```python
from build123d import *

# Parameters (mm, degrees)
F0_W     = 910
F0_H     = 1270
F1_DEPTH = 890
F2_W     = 950
F2_H     = 380
F3_DEPTH = 610
F4_W     = 160
F4_H     = 190
F5_DEPTH = 610


with BuildPart() as f1:
    # F0 (on Top) → F1 (new body)
    with BuildSketch(Plane.XY):
        with Locations((10.50148, 0)):
            Rectangle(F0_W, F0_H)
    extrude(amount=F1_DEPTH)

    # F2 (on face) → F3 (cut)
    with BuildSketch(Plane(origin=(-444.49852, 0, 0), x_dir=(0, -1, 0), z_dir=(-1, 0, 0))):
        with Locations((0, 700)):
            Rectangle(F2_W, F2_H)
    extrude(amount=-F3_DEPTH, mode=Mode.SUBTRACT)

    # F4 (on face) → F5 (cut, through all)
    with BuildSketch(Plane(origin=(-444.49852, 0, 0), x_dir=(0, -1, 0), z_dir=(-1, 0, 0))):
        with Locations((-555, 795)):
            Rectangle(F4_W, F4_H)
        with Locations((555, 795)):
            Rectangle(F4_W, F4_H)
    extrude(amount=-F5_DEPTH, mode=Mode.SUBTRACT)


solid = f1.part
```
Check sheet for the modelled part. Datum: model origin and axes. Units: mm. A direction names the side the tool comes from. Give positions to 0.01 mm unless a question says otherwise; leave off trailing zeros. Write each loop counter-clockwise with the first axis right and the second up, starting at its lowest first coordinate (ties: lowest second). Pieces come first, ordered by that corner, then holes.
Item 1: Cross-section at B-B (x = 23). Enter the section's corners in (y, z), and give its area (4 significant figures).
Item 2: Draft check along Y on faces 1 (the face through (465.501, -9, 439)), 2 (the face through (4, 635, 340)), 3 (the face through (-144, 475, 604)). Enter one of: released by +Y, released by -Y, zero draft, split by the parting line, or undercut.
Item 3: Cross-section at A-A (z = 670.5). Enter the section's corners in (x, y), and give its area (3 significant figures).
Item 4: Scan lines: L1, parallel to Z at x = -226.5, y = 109.5; L2, parallel to X at y = -56, z = 611.5; L3, parallel to Y at x = -393.5, z = 545. Record each from-to range of solid material in increasing order.
Item 5: Access from +Z, -Z, +X, -X, +Y, -Y to the whole of each face (thin tool, end or side, straight path). Record for faces 4 (the face through (4, 9, 0)), 5 (the face through (-144, -475, 604)), 6 (the face through (-144, 556, 700)).
Item 6: Cross-section at C-C (y = 324). Enter the section's corners in (x, z).
Item 7: Cross-section at D-D (z = 787). Enter the section's corners in (x, y), and give its area (3 significant figures).
Report:
1. outline: (-635, 0) - (635, 0) - (635, 700) - (475, 700) - (475, 510) - (-475, 510) - (-475, 700) - (-635, 700) - close
1. area: 708,500 mm2
2. face 1: zero draft
2. face 2: released by +Y
2. face 3: undercut
3. outline: (-444.5, -635) - (465.5, -635) - (465.5, 635) - (-444.5, 635) - (-444.5, 475) - (165.5, 475) - (165.5, -475) - (-444.5, -475) - close
3. area: 576,000 mm2
4. L1: z = 0 to 510
4. L2: x = 165.5 to 465.5
4. L3: y = -635 to -475, 475 to 635
5. face 4: -Z, +X, -X, +Y, -Y
5. face 5: +Z, -X
5. face 6: +Z, -X, +Y, -Y
6. outline: (-444.5, 0) - (465.5, 0) - (465.5, 890) - (165.5, 890) - (165.5, 510) - (-444.5, 510) - close
7. outline: (165.5, -635) - (465.5, -635) - (465.5, 635) - (165.5, 635) - close
7. area: 381,000 mm2
